```python
from build123d import *

# Parameters (mm, degrees)
SKETCH1_W           = 13
SKETCH1_H           = 25
BOSS_EXTRUDE1_DEPTH = 6
SKETCH2_W           = 13
SKETCH2_H           = 25
BOSS_EXTRUDE2_DEPTH = 4
CUT_EXTRUDE1_DEPTH  = 2.5
BOSS_EXTRUDE3_DEPTH = 41
CUT_EXTRUDE2_DEPTH  = 18
FILLET2_R           = 4
FILLET3_R           = 4


with BuildPart() as part:
    # Sketch1 → Boss-Extrude1 (new body)
    with BuildSketch(Plane(origin=(0, 0, 0), x_dir=(1, 0, 0), z_dir=(0, 1, 0))):
        with Locations((6.5, -12.5)):
            Rectangle(SKETCH1_W, SKETCH1_H)
    extrude(amount=BOSS_EXTRUDE1_DEPTH)

    # Sketch3 → Cut-Extrude1 (cut)
    with BuildSketch(Plane(origin=(0, 6, 0), x_dir=(1, 0, 0), z_dir=(0, 1, 0))):
        with BuildLine():
            Line((4.25, -5.207729985), (3.192810861, -15.75))
            ThreePointArc((3.192810861, -15.75), (6.5, -14), (9.807189139, -15.75))
            Line((9.807189139, -15.75), (8.75, -5.207729985))
            ThreePointArc((8.75, -5.207729985), (6.5, -2.957729985), (4.25, -5.207729985))
        make_face()
        with BuildLine():
            ThreePointArc((9.807189139, -15.75), (6.5, -14), (3.192810861, -15.75))
            Line((3.192810861, -15.75), (3.192810861, -20.25))
            ThreePointArc((3.192810861, -20.25), (6.5, -22), (9.807189139, -20.25))
            Line((9.807189139, -20.25), (9.807189139, -15.75))
        make_face()
        with BuildLine():
            Line((3.192810861, -20.25), (3.192810861, -15.75))
            ThreePointArc((3.192810861, -15.75), (2.5, -18), (3.192810861, -20.25))
        make_face()
        with BuildLine():
            ThreePointArc((10.5, -18), (10.322875656, -16.822875656), (9.807189139, -15.75))
            Line((9.807189139, -15.75), (9.807189139, -20.25))
            ThreePointArc((9.807189139, -20.25), (10.322875656, -19.177124344), (10.5, -18))
        make_face()
    extrude(amount=-CUT_EXTRUDE1_DEPTH, mode=Mode.SUBTRACT)



with BuildPart() as body_2:
    # Sketch2 → Boss-Extrude2 (new body)
    with BuildSketch(Plane(origin=(0, 37, 0), x_dir=(1, 0, 0), z_dir=(0, 1, 0))):
        with Locations((6.5, -12.5)):
            Rectangle(SKETCH2_W, SKETCH2_H)
    extrude(amount=BOSS_EXTRUDE2_DEPTH)


with BuildPart() as part_1:
    add(part.part)

    add(body_2.part)  # Boss-Extrude3 merges body 2
    # Sketch4 → Boss-Extrude3 (add, through all)
    with BuildSketch(Plane.XZ):
        with BuildLine():
            Line((-17.376544105, -22.043835706), (-11.894619464, -30.983507581))
            ThreePointArc((-11.894619464, -30.983507581), (5.405335132, -19.390755444), (13, 0))
            Line((13, 0), (0, 0))
            ThreePointArc((0, 0), (-4.675917284, -14.184745799), (-17.376544105, -22.043835706))
        make_face()
    extrude(amount=-BOSS_EXTRUDE3_DEPTH)

    # Sketch5 → Cut-Extrude2 (cut)
    with BuildSketch(Plane(origin=(0, 9, 0), x_dir=(-1, 0, 0), z_dir=(0, -1, 0))):
        with BuildLine():
            Line((1.720669879, 26.072760653), (7.3010615, 16.972513332))
            ThreePointArc((7.3010615, 16.972513332), (12.005611012, 20.170145468), (17.376544105, 22.043835706))
            Line((17.376544105, 22.043835706), (11.894619464, 30.983507581))
            ThreePointArc((11.894619464, 30.983507581), (6.607240555, 28.943325821), (1.720669879, 26.072760653))
        make_face()
    extrude(amount=-CUT_EXTRUDE2_DEPTH, mode=Mode.SUBTRACT)

    # Fillet2
    fillet2_edges = [part_1.edges().sort_by_distance(p)[0] for p in [
        (-17.376544105, 34, -22.043835706),
        (-11.894619464, 34, -30.983507581),
        (-17.376544105, 4.5, -22.043835706),
        (-11.894619464, 4.5, -30.983507581),
    ]]
    fillet(fillet2_edges, radius=FILLET2_R)

    # Fillet3
    fillet3_edges = [part_1.edges().sort_by_distance(p)[0] for p in [
        (0, 3, 25),
        (13, 3, 25),
        (13, 39, 25),
        (0, 39, 25),
    ]]
    fillet(fillet3_edges, radius=FILLET3_R)


solid = part_1.part
```
Model file for the job. Use its own axes, mm. A direction names the side the tool comes from. Give positions to 0.01 mm unless a question says otherwise; leave off trailing zeros. Loops run counter-clockwise (first coordinate to the right, second up) from the corner with the lowest first, then second, coordinate; pieces in that order, holes last. Notation, with made-up numbers: (84, 80) -> (114, 80) arc R27 cw to (114, 110) -> close; hole circle Ø1 at (22.25, 54). An arc over 180 degrees is marked (long way). Use CSV: the item, a comma, the result in double quotes. Start each with the question number.
1) Slice it at C-C on z = -19. Give the cut face in (x, y).
2) Tool access for faces 1 (the flat face through (0, 3, 11)), 2 (the cylindrical face through (11.859, 39.028, 23.797)), 3 (the flat face through (-4.47, 17.87, -21.59)), 4 (the cylindrical face through (6.55, 4.77, 2.96)): list every direction of +Z, -Z, +X, -X, +Y, -Y with a clear straight run to the whole face (end or side of a thin tool).
3) Slice it at A-A on y = 28.5. Give the cut face in (x, z).
4) Mould opens along X. For faces 5 (the flat face through (3.5, 6, 9.5)), 6 (the flat face through (6, 3.5, 14)), 7 (the flat face through (-14.16, 4.44, -27.29)) say: released by +X, released by -X, zero draft, split by the parting line, or undercut.
5) Wall check: line 1 (Y direction, x = 3, z = 10); line 2 (Y direction, x = 5.75, z = 6); line 3 (Z direction, x = 5, y = 14). Give the ranges that are in metal, low to high.
6) Flat gauge pins, fed straight in: pin 1 Ø2 at (y, z) = (20.5, -13.5) entering from +X; pin 2 Ø1.5 at (x, y) = (8.5, 22) entering from +Z; pin 3 Ø3 at (y, z) = (2, 15.5) entering from -X. Where does each tip first touch, or does it go through?
7) Slice it at D-D on y = 38. Give the cut face in (x, z), plus the area to 3 significant figures.
8) Slice it at B-B on x = 6.75. Give the cut face in (y, z), plus the area to 3 significant figures.
Computed values:
1,outline,"(-9.96, 0) -> (5.71, 0) -> (5.71, 41) -> (-9.96, 41) -> (-9.96, 27) -> (-6.06, 27) -> (-6.06, 9) -> (-9.96, 9) -> close"
2,face 1,"+Z, -X, +Y, -Y"
2,face 2,"+Z, +X, +Y, -Y"
2,face 3,"-Z, -X"
2,face 4,"none"
3,outline,"(-14.73, -26.36) -> (-13.58, -28.24) arc R4 ccw to (-8.66, -29.86) arc R34.83 ccw to (13, 0) -> (0, 0) arc R21.83 cw to (-12.95, -20.62) arc R4 ccw to start"
4,face 5,"zero draft"
4,face 6,"undercut"
4,face 7,"released by -X"
5,line 1,"y = 0 to 6, 37 to 41"
5,line 2,"y = 0 to 3.5, 37 to 41"
5,line 3,"z = -19.89 to 0"
6,pin 1,"stops at x = 9.72"
6,pin 2,"stops at z = 0"
6,pin 3,"stops at x = 0"
7,outline,"(-14.73, -26.36) -> (-13.58, -28.24) arc R4 ccw to (-8.66, -29.86) arc R34.83 ccw to (13, 0) -> (13, 21) arc R4 ccw to (9, 25) -> (4, 25) arc R4 ccw to (0, 21) -> (0, 0) arc R21.83 cw to (-12.95, -20.62) arc R4 ccw to start"
7,area,"720 mm^2"
8,outline,"(0, -17.6) -> (41, -17.6) -> (41, 25) -> (37, 25) -> (37, 0) -> (6, 0) -> (6, 2.97) -> (3.5, 2.97) -> (3.5, 21.99) -> (6, 21.99) -> (6, 25) -> (0, 25) -> close"
8,area,"924 mm^2"
